Geometry: final body of the model. Coordinates: model frame, mm. A direction names the side the tool comes from. Round coordinates to 2 decimals unless told otherwise and drop trailing zeros. Loops run counter-clockwise (first coordinate to the right, second up) from the corner with the lowest first, then second, coordinate; pieces in that order, holes last. Notation, with made-up numbers: (42.25, -12) - (84.25, -12) arc R18 cw to (84.25, 7) - close; hole circle Ø7 at (18.5, 36.5). An arc over 180 degrees is marked (long way). Answer as CSV lines item,"result".
from build123d import *

# Parameters (mm, degrees)
SKETCH_1_W          = 20
SKETCH_1_H          = 28.9
EXTRUDE_1_DEPTH     = 7
CUT_EXTRUDE_1_DEPTH = 30.5
SKETCH_3_R          = 1.5
CUT_EXTRUDE_2_DEPTH = 2.5


with BuildPart() as part:
    # 草图1 → 凸台-拉伸1 (new body)
    with BuildSketch(Plane.XY):
        with Locations((-30.686463881, 21.553540909)):
            Rectangle(SKETCH_1_W, SKETCH_1_H)
    extrude(amount=EXTRUDE_1_DEPTH)

    # 草图2 → 切除-拉伸1 (cut)
    with BuildSketch(Plane(origin=(0, 36.003540909, 0), x_dir=(1, 0, 0), z_dir=(0, 1, 0))):
        Polygon((-30.686463881, -7), (-35.686463881, -7), (-35.686463881, -3.5), (-25.686463881, -3.5), (-25.686463881, -7), align=None)
    extrude(amount=-CUT_EXTRUDE_1_DEPTH, mode=Mode.SUBTRACT)

    # 草图3 → 切除-拉伸2 (cut)
    with BuildSketch(Plane(origin=(0, 0, 0), x_dir=(-1, 0, 0), z_dir=(0, 0, -1))):
        with Locations((23.186463881, 31.003540909)):
            Circle(SKETCH_3_R)
        with Locations((38.186463881, 31.003540909)):
            Circle(SKETCH_3_R)
        with Locations((38.186463881, 12.103540909)):
            Circle(SKETCH_3_R)
        with Locations((23.186463881, 12.103540909)):
            Circle(SKETCH_3_R)
    extrude(amount=-CUT_EXTRUDE_2_DEPTH, mode=Mode.SUBTRACT)


solid = part.part
(1) Material intervals for line 1 along X through (y, z) = (19.75, 5.75); line 2 along Z through (x, y) = (-29, 17.25); line 3 along Z through (x, y) = (-24, 31), sorted ascending.
Findings below:
line 1,"-40.69 to -35.69, -25.69 to -20.69"
line 2,"0 to 3.5"
line 3,"2.5 to 7"
(2) Section D-D (x = -37.25). Output: boundary loops of the cut face in (y, z).
Findings below:
outline,"(7.1, 0) - (10.93, 0) - (10.93, 2.5) - (13.28, 2.5) - (13.28, 0) - (29.83, 0) - (29.83, 2.5) - (32.18, 2.5) - (32.18, 0) - (36, 0) - (36, 7) - (7.1, 7) - close"
(3) Access query for faces 5 (the face through (-25.686, 22, 5)), 6 (the face through (-31, 7.104, 3)), 7 (the face through (-39.6, 12.6, 1.2)). Directions: +Z, -Z, +X, -X, +Y, -Y. A direction counts if a zero-diameter tool reaches every point of the face in a straight line with its end or side. Return the directions, or none.
Findings below:
face 5,"+Z, +Y, -Y"
face 6,"+Z, -Z, +X, -X, -Y"
face 7,"-Z"
(4) Pin query (flat end, axial travel): P1, Ø1, axis at x = -30, z = 4.5, coming from the +Y side; P2, Ø1.5, axis at x = -23.5, y = 30.5, coming from the -Z side. Return the tip coordinate at first contact, or that it passes through.
Findings below:
P1,"through"
P2,"z = 2.5"
(5) Section B-B (y = 14.75). Output: boundary loops of the cut face in (x, z).
Findings below:
outline,"(-40.69, 0) - (-20.69, 0) - (-20.69, 7) - (-25.69, 7) - (-25.69, 3.5) - (-35.69, 3.5) - (-35.69, 7) - (-40.69, 7) - close"
(6) Draft query along X for faces 1 (the face through (-20.686, 21, 3)), 2 (the face through (-22.99, 13.59, 1.23)), 3 (the face through (-23, 22, 7)), 4 (the face through (-40.686, 21, 3)). Return one class per face: pulls with the +X half, pulls with the -X half, needs draft (parallel to the pull), parting line crosses it, or undercut.
Findings below:
face 1,"pulls with the +X half"
face 2,"undercut"
face 3,"needs draft"
face 4,"pulls with the -X half"
(7) Section C-C (z = 1.5). Output: boundary loops of the cut face in (x, y).
Findings below:
outline,"(-40.69, 7.1) - (-20.69, 7.1) - (-20.69, 36) - (-40.69, 36) - close; hole circle Ø3 at (-38.19, 12.1); hole circle Ø3 at (-38.19, 31); hole circle Ø3 at (-23.19, 12.1); hole circle Ø3 at (-23.19, 31)"
(8) Section A-A (z = 6.25). Output: boundary loops of the cut face in (x, y), and give its area (3 significant figures).
Findings below:
outline,"(-40.69, 7.1) - (-35.69, 7.1) - (-35.69, 36) - (-40.69, 36) - close; (-25.69, 7.1) - (-20.69, 7.1) - (-20.69, 36) - (-25.69, 36) - close"
area,"289 mm2"
